```python
from build123d import *

# Parameters (mm, degrees)
ESQUISSE1_W        = 75
ESQUISSE1_H        = 71
ESQUISSE1_R        = 1.5
BOSS_EXTRU_1_DEPTH = 2
ESQUISSE3_R        = 12.5
BOSS_EXTRU_2_DEPTH = 32
CONG_1_R           = 3


with BuildPart() as part:
    # Esquisse1 → Boss.-Extru.1 (new body)
    with BuildSketch(Plane(origin=(0, 0, 0), x_dir=(1, 0, 0), z_dir=(0, 1, 0))):
        with Locations((0, -0.5)):
            Rectangle(ESQUISSE1_W, ESQUISSE1_H)
        with Locations((-31.5, 30)):
            Circle(ESQUISSE1_R, mode=Mode.SUBTRACT)
        with Locations((-31.5, -31)):
            Circle(ESQUISSE1_R, mode=Mode.SUBTRACT)
        with Locations((30.5, -1)):
            Circle(ESQUISSE1_R, mode=Mode.SUBTRACT)
    extrude(amount=BOSS_EXTRU_1_DEPTH)

    # Esquisse3 → Boss.-Extru.2 (add)
    with BuildSketch(Plane(origin=(0, 2, 0), x_dir=(1, 0, 0), z_dir=(0, 1, 0))):
        with Locations((-17.5, 20)):
            Circle(ESQUISSE3_R)
    extrude(amount=BOSS_EXTRU_2_DEPTH)

    # Congé1
    cong_1_edges = [part.edges().sort_by_distance(p)[0] for p in [
        (-30, 34, -20),
    ]]
    fillet(cong_1_edges, radius=CONG_1_R)


solid = part.part
```
The model under review builds one solid part; all positions refer to its coordinate system, in mm. A direction names the side the tool comes from. Round coordinates to 2 decimals unless told otherwise and drop trailing zeros. Write each loop counter-clockwise with the first axis right and the second up, starting at its lowest first coordinate (ties: lowest second). Pieces come first, ordered by that corner, then holes. Notation, with made-up numbers: M 29,-5.75 L 51,-5.75 A21 cw 51,8.25 Z; hole C 0.5,47 d3. An arc over 180 degrees is marked long. Use CSV: the item, a comma, the result in double quotes. Start each with the question number.
(1) Clearance check with flat-ended pins moving along their axes: P1, Ø1.5, axis at x = -7, y = 4.5, coming from the -Z side; P2, Ø6, axis at x = 24.5, z = 11.5, coming from the +Y side; P3, Ø6, axis at x = 3.5, z = -12.5, coming from the -Y side; P4, Ø1, axis at y = 22, z = -23, coming from the +X side. State where each tip first meets the part, or that it passes through.
(2) We need section B-B, the plane z = 31. State the section outline as (x, y) points.
(3) For line 1 along Z through (x, y) = (-31.5, 1.05); line 2 along X through (y, z) = (1.15, 1); line 3 along Z through (x, y) = (30.5, 1.4), list the stretches that pass through material, from the lowest coordinate up.
(4) We need section C-C, the plane x = -31.5. State the section outline as (y, z) points.
(5) Tool access review of faces 1 (the face through (-27.42, 16.297, -12.394)), 2 (the face through (-32.61, 0.99, 29.99)): name each direction out of +Z, -Z, +X, -X, +Y, -Y from which nothing blocks a thin tool from reaching the whole face with its end or side.
(6) We need section D-D, the plane z = -20. State the section outline as (x, y) points.
(7) The part is to be moulded in two halves that separate along Z. For faces 3 (the face through (37.5, 1, 1)), 4 (the face through (-1, 1, 36)), 5 (the face through (-32.61, 0.99, -31.01)), say which applies: +Z half, -Z half, draft (parallel to the pull), parting line (faces both ways), or undercut.
(8) We need section A-A, the plane x = 30.5. State the section outline as (y, z) points, then the cut area to 3 significant figures.
Findings:
1,P1,"z = -27.82"
1,P2,"y = 2"
1,P3,"y = 0"
1,P4,"x = -5.25"
2,outline,"M -37.5,0 L -33,0 L -33,2 L -37.5,2 Z; M -30,0 L 37.5,0 L 37.5,2 L -30,2 Z"
3,line 1,"-35 to -31.5, -28.5 to 29.5, 32.5 to 36"
3,line 2,"-37.5 to 29, 32 to 37.5"
3,line 3,"-35 to -0.5, 2.5 to 36"
4,outline,"M 0,-35 L 2,-35 L 2,-31.5 L 0,-31.5 Z; M 0,-28.5 L 2,-28.5 L 2,29.5 L 0,29.5 Z; M 0,32.5 L 2,32.5 L 2,36 L 0,36 Z"
5,face 1,"+Y"
5,face 2,"+Y, -Y"
6,outline,"M -37.5,0 L 37.5,0 L 37.5,2 L -5,2 L -5,31 A3 ccw -8,34 L -27,34 A3 ccw -30,31 L -30,2 L -37.5,2 Z"
7,face 3,"draft"
7,face 4,"+Z half"
7,face 5,"undercut"
8,outline,"M 0,-35 L 2,-35 L 2,-0.5 L 0,-0.5 Z; M 0,2.5 L 2,2.5 L 2,36 L 0,36 Z"
8,area,"136 mm^2"
